from build123d import *

# Parameters (mm, degrees)
F0_W          = 25
F0_H          = 25
F1_DEPTH      = 400
F1_DEPTH_BACK = 400
F2_R          = 4.75
F5_W          = 25
F5_H          = 25
F6_DEPTH      = 300
F7_W          = 25
F7_H          = 25
F7_H_2        = 50
F8_DEPTH      = 5
F9_W          = 25
F9_H          = 25
F10_DEPTH     = 425
F11_W         = 25
F11_H         = 25
F12_DEPTH     = 750
F13_W         = 5
F13_H         = 200
F13_R         = 4.75
F14_DEPTH     = 750
F16_D         = 8.8


with BuildPart() as f1:
    # F0 (on Right) → F1 (new body, two sides)
    with BuildSketch(Plane.YZ) as f1_sk:
        Rectangle(F0_W, F0_H)
    extrude(amount=F1_DEPTH)
    extrude(f1_sk.sketch, amount=-F1_DEPTH_BACK)

    # F4: sweep along a path in F3
    with BuildLine(Plane.YZ) as f4_path:
        Line((-12.5, 0), (-262.5, 0))
        ThreePointArc((-262.5, 0), (-277.7069063257, 1.2585620455), (-292.5, 5))
    # F2 (on face) → F4 (sweep)
    with BuildSketch(Plane.XZ.offset(12.5)):
        with Locations((-100, 0)):
            Circle(F2_R)
        with Locations((100, 0)):
            Circle(F2_R)
        with Locations((-300, 0)):
            Circle(F2_R)
        with Locations((300, 0)):
            Circle(F2_R)
    sweep(path=f4_path.line)

    # F5 (on face) → F6 (join)
    with BuildSketch(Plane(origin=(0, 0, -12.5), x_dir=(1, 0, 0), z_dir=(0, 0, -1))):
        with Locations((-387.5, 0)):
            Rectangle(F5_W, F5_H)
        with Locations((387.5, 0)):
            Rectangle(F5_W, F5_H)
    extrude(amount=F6_DEPTH)

    # F7 (on face) → F8 (join)
    with BuildSketch(Plane(origin=(0, 0, -312.5), x_dir=(1, 0, 0), z_dir=(0, 0, -1))):
        with Locations((-387.5, 0)):
            Rectangle(F7_W, F7_H)
        with Locations((-387.5, -37.5)):
            Rectangle(F7_W, F7_H_2)
        with Locations((-387.5, 37.5)):
            Rectangle(F7_W, F7_H_2)
        with Locations((387.5, 0)):
            Rectangle(F7_W, F7_H)
        with Locations((387.5, 37.5)):
            Rectangle(F7_W, F7_H_2)
        with Locations((387.5, -37.5)):
            Rectangle(F7_W, F7_H_2)
    extrude(amount=F8_DEPTH)

    # F9 (on face) → F10 (join)
    with BuildSketch(Plane.XY.offset(12.5)):
        with Locations((-387.5, 0)):
            Rectangle(F9_W, F9_H)
        with Locations((387.5, 0)):
            Rectangle(F9_W, F9_H)
    extrude(amount=F10_DEPTH)

    # F11 (on face) → F12 (join, through all)
    with BuildSketch(Plane.YZ.offset(-375)):
        with Locations((0, 425)):
            Rectangle(F11_W, F11_H)
    extrude(amount=F12_DEPTH)

    # F13 (on face) → F14 (join, through all)
    with BuildSketch(Plane.YZ.offset(-375)):
        with Locations((0, 112.5)):
            Rectangle(F13_W, F13_H)
        with Locations((0, 372.5)):
            Circle(F13_R)
        with Locations((0, 332.5)):
            Circle(F13_R)
        with Locations((0, 292.5)):
            Circle(F13_R)
        with Locations((0, 252.5)):
            Circle(F13_R)
    extrude(amount=F14_DEPTH)

    # F16 (through all)
    with Locations(Plane.XY.offset(-312.5)):
        with Locations((-387.5, -37.5), (-387.5, 37.5), (387.5, -37.5), (387.5, 37.5)):
            Hole(F16_D / 2)


solid = f1.part
Source: CAD feature listing. Evaluate the final solid. Frame: model axes, mm. A direction names the side the tool comes from. Round coordinates to 2 decimals unless told otherwise and drop trailing zeros. Order: outer loops, then holes, each group sorted by start corner. A loop starts at its lowest first (then second) coordinate and runs counter-clockwise, first axis right, second up. Notation, with made-up numbers: (-29, 3) -> (1, 3) arc R18 cw to (1, 16) -> close; hole circle Ø10 at (-19.5, 86.5). An arc over 180 degrees is marked (long way). Answer as CSV lines item,"result".
Item 1: Line query: L1, parallel to Z at x = 214.5, y = 1; L2, parallel to Y at x = -387, z = -314; L3, parallel to X at y = -37, z = -313. Output: solid intervals per line, ascending.
A:
L1,"-12.5 to 212.5, 247.86 to 257.14, 287.86 to 297.14, 327.86 to 337.14, 367.86 to 377.14, 412.5 to 437.5"
L2,"-62.5 to -41.87, -33.13 to 33.13, 41.87 to 62.5"
L3,"-400 to -391.87, -383.13 to -375, 375 to 383.13, 391.87 to 400"
Item 2: Pin query (flat end, axial travel): pin 1 Ø7.5 at (x, y) = (382.5, 43) entering from +Z; pin 2 Ø2.5 at (x, z) = (-385.5, -316) entering from -Y; pin 3 Ø7.5 at (x, y) = (80, 1.5) entering from -Z; pin 4 Ø7 at (x, y) = (387.5, -37.5) entering from -Z. Return the tip coordinate at first contact, or that it passes through.
A:
pin 1,"z = -312.5"
pin 2,"y = -62.5"
pin 3,"z = -12.5"
pin 4,"through"
Item 3: Reachability of faces 1 (the face through (-5, 2.5, 111)), 2 (the face through (375, 0, -164)), 3 (the face through (-5, 0, 412.5)) from +Z, -Z, +X, -X, +Y, -Y: full face, straight path, thin tool, end or side. Return the list, or none.
A:
face 1,"+Y"
face 2,"-Z, +Y, -Y"
face 3,"+Y, -Y"
Item 4: Section C-C, the plane y = -190.5. Return loops of the section in (x, z).
A:
outline,"circle Ø9.5 at (-300, 0); circle Ø9.5 at (-100, 0); circle Ø9.5 at (100, 0); circle Ø9.5 at (300, 0)"
Item 5: Pull-direction query (Z, two-part tool) for faces 4 (the face through (-400, 0, 58)), 5 (the face through (-375, -3, 210)), 6 (the face through (-6, 0, 437.5)); classes: pulls with the +Z half, pulls with the -Z half, needs draft (parallel to the pull), parting line crosses it, or undercut.
A:
face 4,"needs draft"
face 5,"undercut"
face 6,"pulls with the +Z half"
Item 6: Section A-A, the plane x = 116.5. Return loops of the section in (y, z), plus the area to 3 significant figures.
A:
outline,"(-12.5, -12.5) -> (12.5, -12.5) -> (12.5, 12.5) -> (2.5, 12.5) -> (2.5, 212.5) -> (-2.5, 212.5) -> (-2.5, 12.5) -> (-12.5, 12.5) -> close; (-12.5, 412.5) -> (12.5, 412.5) -> (12.5, 437.5) -> (-12.5, 437.5) -> close; circle Ø9.5 at (0, 252.5); circle Ø9.5 at (0, 292.5); circle Ø9.5 at (0, 332.5); circle Ø9.5 at (0, 372.5)"
area,"2,530 mm²"
Item 7: Section B-B, the plane z = -73. Return loops of the section in (x, y).
A:
outline,"(-400, -12.5) -> (-375, -12.5) -> (-375, 12.5) -> (-400, 12.5) -> close; (375, -12.5) -> (400, -12.5) -> (400, 12.5) -> (375, 12.5) -> close"
